Can you work these out from the model? Positions are in its coordinate system, mm. A direction names the side the tool comes from. Round coordinates to 2 decimals unless told otherwise and drop trailing zeros. Order: outer loops, then holes, each group sorted by start corner. A loop starts at its lowest first (then second) coordinate and runs counter-clockwise, first axis right, second up. Notation, with made-up numbers: (-22.5, 77) - (8.5, 77) arc R21 ccw to (8.5, 85) - close; hole circle Ø6 at (-4.5, 82). An arc over 180 degrees is marked (long way). Write item = value, one per line.
Autodesk Inventor part; units mm, degrees
ref_plane "YZ Plane" through (0, 0, 0) normal (1, 0, 0) x (0, 1, 0)
ref_plane "XZ Plane" through (0, 0, 0) normal (0, 1, 0) x (-1, 0, 0)
ref_plane "XY Plane" through (0, 0, 0) normal (0, 0, 1) x (1, 0, 0)
sketch "Sketch1" plane through (0, 0, 0) normal (0, 1, 0) x (-1, 0, 0)
  circle A0 centre (0, 0) radius 4.5
  dimension "d0" = 9
extrude "Extrusion1" add sketch "Sketch1" along normal blind 5
sketch "Sketch2" plane through (0, 5, 0) normal (0, 1, 0) x (1, 0, 0)
  circle A0 centre (0, 0) radius 4.5
  line L0 (0, 0) -> (-1, 0)
  line L1 (-1, 0) -> (1, 0)
  line L2 (1, 0) -> (1, 8.5977)
  line L3 (1, 8.5977) -> (-1, 8.5977)
  line L4 (-1, 8.5977) -> (-1, -7.4697)
  line L5 (-1, -7.4697) -> (1, -7.4697)
  line L6 (1, -7.4697) -> (1, 8.5977)
  dimension "d4" = 1
  dimension "d5" = 2
extrude "Extrusion2" add sketch "Sketch2" along normal blind 5 contours L2 L1 L0 L4 A0 | A0 L4 L3 L2 | L6 L5 L4 A0 | A0 L4 L0 L1 L6
sketch "Sketch3" plane through (0, 5, 0) normal (0, -1, 0) x (1, 0, 0)
  arc A0 (1, 4.3875) -> (-1, 4.3875) centre (0, 0) ccw
  line L0 (1, 7.4697) -> (1, 4.3875)
  line L1 (-1, 7.4697) -> (1, 7.4697)
  line L2 (-1, 4.3875) -> (-1, 7.4697)
  arc A1 (-1, -4.3875) -> (1, -4.3875) centre (0, 0) ccw
  line L3 (-1, -8.5977) -> (-1, -4.3875)
  line L4 (1, -8.5977) -> (-1, -8.5977)
  line L5 (1, -4.3875) -> (1, -8.5977)
extrude "Extrusion3" cut sketch "Sketch3" against normal blind 5
sketch "Sketch7" plane through (1, 5, 4.3875) normal (1, 0, 0) x (0, 0, -1)
  line L0 (4.3875, 2) -> (4.3875, 1)
  circle A0 centre (4.3875, 1) radius 2
  point P0 (4.3875, -5)
  dimension "d20" = 1
  dimension "d21" = 4
extrude "Extrusion7" cut sketch "Sketch7" along normal blind 25.4
sketch "Sketch8" plane through (1, 5, -4.3875) normal (1, 0, 0) x (0, 0, -1)
  line L0 (0, 5) -> (-8.775, 5)
  line L1 (0, 5) -> (-8.775, 5)
  line L2 (-8.775, 5) -> (-10.2746, 5)
  line L3 (-10.2746, 5) -> (-10.2746, 3.5)
  line L4 (-10.2746, 3.5) -> (1.1183, 3.5)
  line L5 (1.1183, 3.5) -> (1.1183, 5)
  line L6 (1.1183, 5) -> (0, 5)
  point P0 (-4.3875, -5)
  dimension "d24" = 1.5
extrude "Extrusion8" cut sketch "Sketch8" against normal blind 25.4
fillet "Fillet2" radius 1 2 edges at (0, 8.5, 4.5) (0, 8.5, -4.5)
properties part number "PistonCylinder"
(1) If I drill on line 1 (Y direction, x = -2.5, z = 0.75); line 2 (X direction, y = 5.5, z = 4.25); line 3 (X direction, y = 1.25, z = 1), over which ranges is the centre line in solid material (lowest first)? Write a range as from..to.
Computed:
line_1 = 0..5
line_2 = -1..1
line_3 = -4.39..4.39
(2) On a 3-axis mill with a long thin cutter (end or side, diameter ignored), from which of +Z, -Z, +X, -X, +Y, -Y can I reach the whole of each face in a straight line? I mean faces 1 (the face through (-1, 7, 0)), 2 (the face through (2, 5, 3)), 3 (the face through (3, 4, 0)). Say none if no direction works.
Computed:
face_1 = +Z, -Z, -X, +Y
face_2 = +Z, -Z, +X, +Y
face_3 = +X, +Y
(3) Will these pins go through, and if not, where does the flat tip stop? P1, Ø3, axis at y = 2, z = 2, coming from the -X side; P2, Ø1.3, axis at x = 3, z = -3.5, coming from the +Y side; P3, Ø2.5, axis at y = 7, z = 0.5, coming from the +X side.
Computed:
P1 = -4.47
P2 = 5
P3 = 1
(4) If we section it at B-B (y = 3.5): Write out the boundary of the cut face in (x, z), plus the area to 3 significant figures.
Computed:
outline = circle Ø9 at (0, 0)
area = 63.6 mm^2
(5) If we section it at C-C (x = 1.25): Write out the boundary of the cut face in (y, z), plus the area to 3 significant figures.
Computed:
outline = (0, -4.32) - (5, -4.32) - (5, -1.73) arc R2 cw to (5, 1.73) - (5, 4.32) - (0, 4.32) - close
area = 40.8 mm^2
(6) If we section it at A-A (z = 0): Write out the boundary of the cut face in (x, y).
Computed:
outline = (-4.5, 0) - (4.5, 0) - (4.5, 4) - (1, 4) - (1, 8.5) - (-1, 8.5) - (-1, 5) - (-4.5, 5) - close
(7) If we section it at D-D (y = 5.5): Write out the boundary of the cut face in (x, z), plus the area to 3 significant figures.
Computed:
outline = (-1, -4.39) arc R4.5 ccw to (1, -4.39) - (1, 4.39) arc R4.5 ccw to (-1, 4.39) - close
area = 17.9 mm^2
